Can you work these out from the model? Positions are in its coordinate system, mm. Face numbers are marked on the shaded views. A direction names the side the tool comes from. Coordinates: 2 decimals unless noted, no trailing zeros. Order: outer loops, then holes, each group sorted by start corner. A loop starts at its lowest first (then second) coordinate and runs counter-clockwise, first axis right, second up. Notation, with made-up numbers: (52, 52) -> (61, 52) arc R9 ccw to (61, 56) -> close; hole circle Ø6 at (20, 16). An arc over 180 degrees is marked (long way). Write item = value, one per line.
```python
from build123d import *

# Parameters (mm, degrees)
SKETCH2_R          = 1.905
CUT_EXTRUDE1_DEPTH = 38.1


with BuildPart() as part:
    # Sketch1 → Revolve1 (revolve)
    with BuildSketch(Plane.XY, mode=Mode.PRIVATE) as revolve1_sk:
        Polygon((12.7, 182.88), (27.94, 182.88), (27.94, 157.48), (25.4, 157.48), (25.4, 0), (8.450222624, 0), (8.450222624, -38.1), (0, -38.1), (0, 0), (0, 182.88), (0, 208.28), (12.7, 208.28), align=None)
    revolve(revolve1_sk.sketch.rotate(Axis((0, 0, 0), (0, 1, 0)), 90), axis=Axis((0, 0, 0), (0, 1, 0)))

    # Sketch2 → Cut-Extrude1 (cut)
    with BuildSketch(Plane.XZ.offset(38.1)):
        with Locations(Location((0, 0, 0), (0, 0, 270))):
            Circle(SKETCH2_R)
    extrude(amount=-CUT_EXTRUDE1_DEPTH, mode=Mode.SUBTRACT)


solid = part.part
```
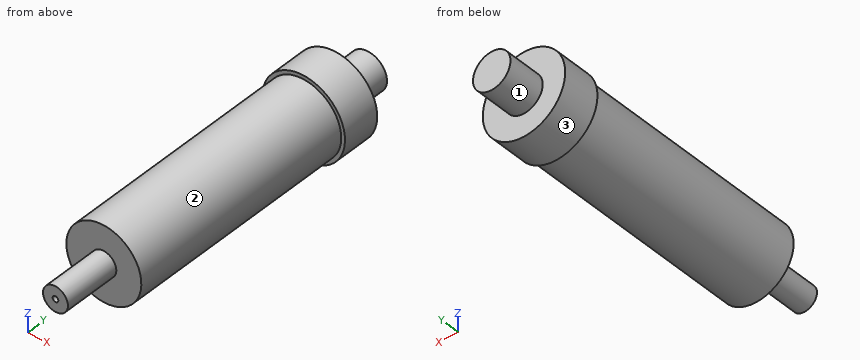
Item 1: For the marked faces 1, 2 and 3, which set-ups out of +Z, -Z, +X, -X, +Y, -Y let a thin tool reach every point of the face, with its end or its side?
A:
face_1 = +Y
face_2 = -Y
face_3 = +Y, -Y
Item 2: I want a section at B-B, the plane y = 20.5. Please give me the cut outline in (x, z).
A:
outline = circle Ø50.8 at (0, 0)
Item 3: I'm going to push flat-ended pins straight in: P1, Ø1.5, axis at y = 160, z = -19.5, coming from the -X side; P2, Ø4, axis at y = 83.5, z = 19, coming from the +X side; P3, Ø2, axis at x = -15, z = 9.5, coming from the -Y side. Where does each tip first touch, or does it pass through?
A:
P1 = -20.71
P2 = 18.87
P3 = 0
Item 4: If I drill on probe 1 along X at (y, z) = (-15, 0) (3 decimals); probe 2 along Y at (x, z) = (-23.5, 10.5); probe 3 along X at (y, z) = (194.5, 1), over which ranges is the centre line in solid material (lowest first)?
A:
probe_1 = -8.45 to -1.905, 1.905 to 8.45
probe_2 = 157.48 to 182.88
probe_3 = -12.66 to 12.66
Item 5: I want a section at C-C, the plane x = -22.5. Please give me the cut outline in (y, z).
A:
outline = (0, -11.79) -> (157.48, -11.79) -> (157.48, -16.56) -> (182.88, -16.56) -> (182.88, 16.56) -> (157.48, 16.56) -> (157.48, 11.79) -> (0, 11.79) -> close
Item 6: I want a section at A-A, the plane z = 21.5. Please give me the cut outline in (x, y).
A:
outline = (-17.84, 157.48) -> (-13.52, 157.48) -> (-13.52, 0) -> (13.52, 0) -> (13.52, 157.48) -> (17.84, 157.48) -> (17.84, 182.88) -> (-17.84, 182.88) -> close
Item 7: I want a section at D-D, the plane z = 5.5. Please give me the cut outline in (x, y).
A:
outline = (-27.39, 157.48) -> (-24.8, 157.48) -> (-24.8, 0) -> (-6.42, 0) -> (-6.42, -38.1) -> (6.42, -38.1) -> (6.42, 0) -> (24.8, 0) -> (24.8, 157.48) -> (27.39, 157.48) -> (27.39, 182.88) -> (11.45, 182.88) -> (11.45, 208.28) -> (-11.45, 208.28) -> (-11.45, 182.88) -> (-27.39, 182.88) -> close
